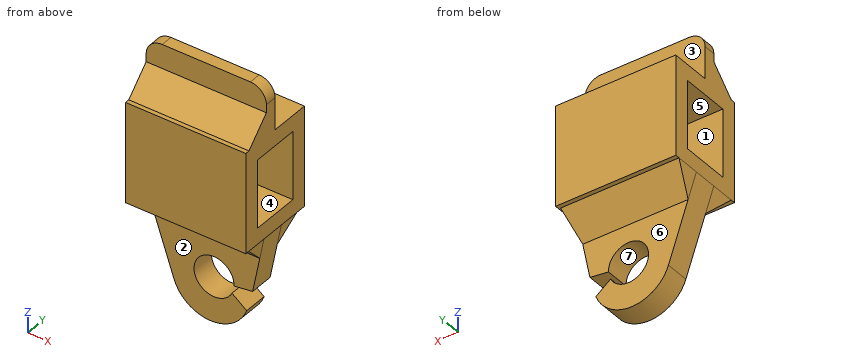
```python
from build123d import *

# Parameters (mm, degrees)
F0_W         = 10.1
F0_H         = 12.5
F0_W_2       = 6.1
F0_H_2       = 8.5
F1_DEPTH     = 15
F3_DEPTH     = 1.5
F5_DEPTH     = 1.5
F6_T1_DEPTH  = 15
F6_T6_DEPTH  = 22.4868112825
F6_T12_DEPTH = 22.4868112825


# Not quite as in the source:
# - a fillet or chamfer that OpenCascade refuses, or shapes differently, is made with other operations: its cross-section is extruded or revolved along the edge and cut away or added


with BuildPart() as f1:
    # F0 (on Right) → F1 (new body)
    with BuildSketch(Plane.YZ):
        Rectangle(F0_W, F0_H)
        Rectangle(F0_W_2, F0_H_2, mode=Mode.SUBTRACT)
    extrude(amount=F1_DEPTH)

    # F2 (on Front) → F3 (join, symmetric)
    with BuildSketch(Plane.XZ):
        with BuildLine():
            Line((14.7717623186, -6.25), (0, -6.25))
            Line((0, -6.25), (3.4864366891, -16.3906378753))
            ThreePointArc((3.4864366891, -16.3906378753), (7.9854016639, -19.6317508441), (12.5416083041, -16.4716115793))
            Line((12.5416083041, -16.4716115793), (10.7079865556, -15.0650723372))
            ThreePointArc((10.7079865556, -15.0650723372), (6.0450329155, -13.3366260518), (10.964385436, -14.0650723372))
            Line((10.964385436, -14.0650723372), (13.2847928678, -13.7592216636))
            Line((13.2847928678, -13.7592216636), (14.7717623186, -6.25))
        make_face()
    extrude(amount=F3_DEPTH, both=True)

    # F4 (on Front) → F5 (join)
    with BuildSketch(Plane.XZ):
        with BuildLine():
            Line((0, 10.25), (0, 6.25))
            Line((0, 6.25), (15, 6.25))
            Line((15, 6.25), (15, 10.25))
            ThreePointArc((15, 10.25), (14.4142135624, 11.6642135624), (13, 12.25))
            Line((13, 12.25), (2, 12.25))
            ThreePointArc((2, 12.25), (0.5857864376, 11.6642135624), (0, 10.25))
        make_face()
    extrude(amount=F5_DEPTH)

    # F6: chamfer of 3 on 3 edges, made by hand

    # F6_s2 → F6_t1 (join)
    with BuildSketch(Plane.YZ):
        Polygon((-4.5, 6.25), (-1.5, 9.25), (-1.5, 6.25), align=None)
    extrude(amount=F6_T1_DEPTH)


with BuildPart() as f6_tool4:
    # F6_s5 → F6_t6 (new body)
    with BuildSketch(Plane.YZ.offset(22.4868112825)):
        Polygon((-4.5, -6.25), (-1.5, -9.25), (-1.5, -6.25), align=None)
    extrude(amount=-F6_T6_DEPTH)

    split(bisect_by=Plane(origin=(15.4053151941, 0, -3.0505469275), x_dir=(0, 1, 0), z_dir=(-0.9809525786, 0, 0.1942473644)), keep=Keep.TOP)

    split(bisect_by=Plane(origin=(-1.9216548906, 0, -0.6606811324), x_dir=(0, 1, 0), z_dir=(0.945669614, 0, 0.3251291761)), keep=Keep.TOP)


with BuildPart() as f1_1:
    add(f1.part)

    # F6_t3: union F6_tool4
    add(f6_tool4.part)


with BuildPart() as f6_tool10:
    # F6_s11 → F6_t12 (new body)
    with BuildSketch(Plane.YZ.offset(22.4868112825)):
        Polygon((4.5, -6.25), (1.5, -9.25), (1.5, -6.25), align=None)
    extrude(amount=-F6_T12_DEPTH)

    split(bisect_by=Plane(origin=(15.4053151941, 0, -3.0505469275), x_dir=(0, 1, 0), z_dir=(-0.9809525786, 0, 0.1942473644)), keep=Keep.TOP)

    split(bisect_by=Plane(origin=(-1.9216548906, 0, -0.6606811324), x_dir=(0, 1, 0), z_dir=(0.945669614, 0, 0.3251291761)), keep=Keep.TOP)


with BuildPart() as f1_2:
    add(f1_1.part)

    # F6_t9: union F6_tool10
    add(f6_tool10.part)


solid = f1_2.part
```
Source: CAD feature listing. Evaluate the final solid. Frame: model axes, mm. Face numbers are marked on the shaded views. A direction names the side the tool comes from. Round coordinates to 2 decimals unless told otherwise and drop trailing zeros. Loops run counter-clockwise (first coordinate to the right, second up) from the corner with the lowest first, then second, coordinate; pieces in that order, holes last.
1. Ray query, L1, parallel to Y at x = 5.5, z = 4; L2, parallel to Y at x = 8, z = 11; L3, parallel to Y at x = 8.25, z = -9.5. Return the intervals inside material, ascending.
2. Section query B-B on z = 3.5. Output: boundary loops of the cut face in (x, y), and give its area (3 significant figures).
3. Section query D-D on x = 5.5. Output: boundary loops of the cut face in (y, z), and give its area (3 significant figures).
4. Section query C-C on x = 8.75. Output: boundary loops of the cut face in (y, z).
5. Access query for the marked faces 1, 2 and 3. Directions: +Z, -Z, +X, -X, +Y, -Y. A direction counts if a zero-diameter tool reaches every point of the face in a straight line with its end or side. Return the directions, or none.
6. Contact query for flat-ended pins moving along their axis: pin 1 (2.5 mm diameter, centred on x = 7, z = 11, fed in from -Y); pin 2 (4 mm diameter, centred on x = 8, y = 2.5, fed in from +Z); pin 3 (1.5 mm diameter, centred on y = 3, z = -8, fed in from +X). Output: stop coordinate, or through.
7. Mould query, pull axis Y, two halves, no side actions, for the marked faces 4, 5, 6 and 7. Classes: released by +Y, released by -Y, zero draft, split by the parting line, or undercut.
8. Section query A-A on y = 1. Output: boundary loops of the cut face in (x, z), and give its area (3 significant figures).
Answers below:
1. L1: y = -5.05 to -3.05, 3.05 to 5.05
1. L2: y = -1.5 to 0
1. L3: y = -1.5 to 1.5
2. outline: (0, -5.05) - (15, -5.05) - (15, -3.05) - (0, -3.05) - close; (0, 3.05) - (15, 3.05) - (15, 5.05) - (0, 5.05) - close
2. area: 60.0 mm2
3. outline: (-5.05, -6.25) - (-4.5, -6.25) - (-1.5, -9.25) - (-1.5, -18.91) - (1.5, -18.91) - (1.5, -9.25) - (4.5, -6.25) - (5.05, -6.25) - (5.05, 6.25) - (0, 6.25) - (0, 12.25) - (-1.5, 12.25) - (-1.5, 9.25) - (-4.5, 6.25) - (-5.05, 6.25) - close; hole (-3.05, -4.25) - (3.05, -4.25) - (3.05, 4.25) - (-3.05, 4.25) - close
3. area: 135 mm2
4. outline: (-5.05, -6.25) - (-4.5, -6.25) - (-1.5, -9.25) - (-1.5, -11.47) - (1.5, -11.47) - (1.5, -9.25) - (4.5, -6.25) - (5.05, -6.25) - (5.05, 6.25) - (0, 6.25) - (0, 12.25) - (-1.5, 12.25) - (-1.5, 9.25) - (-4.5, 6.25) - (-5.05, 6.25) - close; (-1.5, -19.58) - (1.5, -19.58) - (1.5, -16.44) - (-1.5, -16.44) - close; hole (-3.05, -4.25) - (3.05, -4.25) - (3.05, 4.25) - (-3.05, 4.25) - close
5. face 1: +X, -X
5. face 2: -Z, +X, -X, -Y
5. face 3: +Z, +X, -X, +Y
6. pin 1: stops at y = -1.5
6. pin 2: stops at z = 6.25
6. pin 3: stops at x = 14.57
7. face 4: undercut
7. face 5: undercut
7. face 6: released by +Y
7. face 7: zero draft
8. outline: (0, -6.25) - (3.49, -16.39) arc R4.8 ccw to (12.54, -16.47) - (10.71, -15.07) arc R2.5 cw (long way) to (10.96, -14.07) - (13.28, -13.76) - (14.77, -6.25) - (15, -6.25) - (15, -4.25) - (0, -4.25) - close; (0, 4.25) - (15, 4.25) - (15, 6.25) - (0, 6.25) - close
8. area: 179 mm2
